from build123d import *

# Parameters (mm, degrees)
F1_DEPTH = 63.5
F0_W     = 25.2398125172
F0_H     = 19.05
F2_DEPTH = 25.4
F3_DEPTH = 7.9375
F5_R     = 6.35


with BuildPart() as f1:
    # F0 (on Front) → F1 (new body, symmetric)
    with BuildSketch(Plane.XZ):
        Polygon((-41.275, -9.525), (41.275, -9.525), (41.275, 9.525), (22.225, 9.525), (-41.275, 9.525), align=None)
    extrude(amount=F1_DEPTH, both=True)

    # F0 (on Front) → F2 (join, symmetric)
    with BuildSketch(Plane.XZ):
        with Locations((72.9449062586, 52.4002)):
            Rectangle(F0_W, F0_H)
        with BuildLine():
            Line((22.225, 9.525), (41.275, 9.525))
            Line((41.275, 9.525), (41.275, 27.0002))
            ThreePointArc((41.275, 27.0002), (45.9246798487, 38.2255201513), (57.15, 42.8752))
            Line((57.15, 42.8752), (60.325, 42.8752))
            Line((60.325, 42.8752), (60.325, 61.9252))
            Line((60.325, 61.9252), (57.15, 61.9252))
            ThreePointArc((57.15, 61.9252), (32.4542956671, 51.6959043329), (22.225, 27.0002))
            Line((22.225, 27.0002), (22.225, 9.525))
        make_face()
    extrude(amount=F2_DEPTH, both=True)

    # F0 (on Front) → F3 (join, symmetric)
    with BuildSketch(Plane.XZ):
        with BuildLine():
            add(Edge.make_bspline(
                [(-41.275, 9.525), (-42.1492531896, 31.8932123482), (-11.5411048755, 62.5013560057), (57.15, 61.9252)],
                knots=[0, 0, 0, 0, 111.5045361635, 111.5045361635, 111.5045361635, 111.5045361635], degree=3))
            Line((-41.275, 9.525), (22.225, 9.525))
            Line((22.225, 9.525), (22.225, 27.0002))
            ThreePointArc((22.225, 27.0002), (32.4542956671, 51.6959043329), (57.15, 61.9252))
        make_face()
    extrude(amount=F3_DEPTH, both=True)

    # F0 (on Front) → F4 (revolve)
    with BuildSketch(Plane.XZ):
        Polygon((111.125, 66.675), (85.5648125172, 66.675), (85.725, 38.1), (111.125, 38.1), align=None)
    revolve(axis=Axis((85.6449062586, 0, 52.3875), (-0.0056057731, 0, 0.9999842875)))

    # F5
    f5_edges = [f1.edges().sort_by_distance(p)[0] for p in [
        (41.275, 63.5, 0),
        (-41.275, 63.5, 0),
        (-41.275, -63.5, 0),
        (41.275, -63.5, 0),
    ]]
    fillet(f5_edges, radius=F5_R)


solid = f1.part
Input: part model. Units: mm. Frame: model coordinates. A direction names the side the tool comes from. Coordinates: 2 decimals unless noted, no trailing zeros. Loops run counter-clockwise (first coordinate to the right, second up) from the corner with the lowest first, then second, coordinate; pieces in that order, holes last. Notation, with made-up numbers: (-23, 72.5) -> (-5, 72.5) arc R31 ccw to (-5, 96.5) -> close; hole circle Ø11 at (-31.5, -0.75). An arc over 180 degrees is marked (long way). Write each question's results on one line, items separated by ' | '. Start each with the question number.
Q1. Pull-direction query (X, two-part tool) for faces 4 (the flat face through (60, 2, 42.875)), 5 (the flat face through (-3, 7.938, 30)), 6 (the cylindrical face through (39.464, -61.59, 0.133)), 7 (the flat face through (22.225, -17, 18)); classes: released by +X, released by -X, zero draft, split by the parting line, or undercut.
Q2. Pin query (flat end, axial travel): pin 1 (8.5 mm diameter, centred on y = 18, z = 17.5, fed in from -X) (3 decimals); pin 2 (20.5 mm diameter, centred on x = 65.5, y = 6.5, fed in from +Z); pin 3 (9.5 mm diameter, centred on y = 2, z = -5, fed in from -X) (3 decimals). Return the tip coordinate at first contact, or that it passes through.
Q3. Ray query, line 1 (Y direction, x = 60, z = 57); line 2 (X direction, y = 26, z = -4.5) (3 decimals); line 3 (Y direction, x = -10, z = 48). Return the intervals inside material, ascending. Write a range as from..to.
Q4. Section A-A, the plane y = 32. Return the cut outline in (x, z) (3 decimals).
Q5. Reachability of faces 1 (the flat face through (41.275, -1, 4)), 2 (the conical face through (109.95, 7.65, 52.58)), 3 (the flat face through (-3, -7.938, 30)) from +Z, -Z, +X, -X, +Y, -Y: full face, straight path, thin tool, end or side. Return the list, or none.
Found:
1) face 4: undercut | face 5: zero draft | face 6: released by +X | face 7: released by -X
2) pin 1: x = 22.225 | pin 2: z = 66.56 | pin 3: x = -41.275
3) line 1: -25.4..25.4 | line 2: -41.275..41.275 | line 3: -7.94..7.94
4) outline: (-41.275, -9.525) -> (41.275, -9.525) -> (41.275, 9.525) -> (-41.275, 9.525) -> close
5) face 1: -Z, +X, +Y, -Y | face 2: none | face 3: +Z, -X, -Y
